Autodesk Inventor part; units mm, degrees
ref_plane "YZ Plane" through (0, 0, 0) normal (1, 0, 0) x (0, 1, 0)
ref_plane "XZ Plane" through (0, 0, 0) normal (0, 1, 0) x (-1, 0, 0)
ref_plane "XY Plane" through (0, 0, 0) normal (0, 0, 1) x (1, 0, 0)
sketch "Sketch1" plane through (0, 0, 0) normal (0, 1, 0) x (-1, 0, 0)
  line L0 (-10, -55) -> (-160, -55)
  line L1 (-160, -55) -> (-160, -45)
  line L2 (-160, -45) -> (-10, -45)
  line L3 (-10, -45) -> (-10, -55)
  line L4 (10, -55) -> (80, -55)
  line L5 (80, -55) -> (80, -90)
  line L6 (80, -90) -> (110, -90)
  line L7 (110, -90) -> (110, -10)
  line L8 (110, -10) -> (80, -10)
  line L9 (80, -10) -> (80, -45)
  line L10 (80, -45) -> (10, -45)
  line L11 (10, -45) -> (10, -55)
  line L12 (0, -122.2654) -> (0, -189.4683)
  line L13 (-10, 55) -> (-10, 45)
  line L14 (10, 55) -> (10, 45)
  line L15 (80, 10) -> (110, 10)
  line L16 (10, 45) -> (80, 45)
  line L17 (80, 45) -> (80, 10)
  line L18 (80, 55) -> (10, 55)
  line L19 (80, 90) -> (80, 55)
  line L20 (110, 10) -> (110, 90)
  line L21 (110, 90) -> (80, 90)
  line L22 (-160, 55) -> (-10, 55)
  line L23 (-160, 45) -> (-160, 55)
  line L24 (-10, 45) -> (-160, 45)
  point P0 (0, 0)
  dimension "d0" = 10
  dimension "d1" = 80
  dimension "d2" = 10
  dimension "d4" = 30
  dimension "d5" = 30
  dimension "d6" = 35
  dimension "d7" = 35
  dimension "d8" = 45
  dimension "d9" = 10
  dimension "d10" = 10
  dimension "d11" = 150
  dimension "d12" = 100
  dimension "d13" = 0
  dimension "d16" = 100
extrude "Extrusion1" add sketch "Sketch1" along normal blind 50
sketch "Sketch2" plane through (160, 0, 55) normal (1, 0, 0) x (0, 0, -1)
  line L0 (2.5, 40) -> (7.5, 40)
  line L1 (7.5, 40) -> (7.5, 35)
  line L2 (7.5, 35) -> (2.5, 35)
  line L3 (2.5, 35) -> (2.5, 40)
  line L4 (0, 50) -> (10, 50)
  line L5 (10, 0) -> (10, 50)
  line L6 (2.5, 15) -> (7.5, 15)
  line L7 (7.5, 15) -> (7.5, 10)
  line L8 (7.5, 10) -> (2.5, 10)
  line L9 (2.5, 10) -> (2.5, 15)
  line L10 (102.5, 40) -> (107.5, 40)
  line L11 (107.5, 40) -> (107.5, 35)
  line L12 (107.5, 35) -> (102.5, 35)
  line L13 (102.5, 35) -> (102.5, 40)
  line L14 (102.5, 15) -> (107.5, 15)
  line L15 (107.5, 15) -> (107.5, 10)
  line L16 (107.5, 10) -> (102.5, 10)
  line L17 (102.5, 10) -> (102.5, 15)
  point P0 (55, 0)
  dimension "d23" = 10
  dimension "d24" = 5
  dimension "d25" = 2.5
  dimension "d26" = 5
  dimension "d29" = 25
  dimension "d32" = 100
extrude "Extrusion2" cut sketch "Sketch2" against normal blind 200
sketch "Sketch3" plane through (0, 50, 0) normal (0, 1, 0) x (1, 0, 0)
  line L0 (-105, -20) -> (-85, -20)
  line L1 (-85, -20) -> (-85, -30)
  line L2 (-85, -30) -> (-105, -30)
  line L3 (-105, -30) -> (-105, -20)
  line L4 (-110, -10) -> (-110, -90)
  line L5 (-105, -70) -> (-85, -70)
  line L6 (-85, -70) -> (-85, -80)
  line L7 (-85, -80) -> (-105, -80)
  line L8 (-105, -80) -> (-105, -70)
  line L9 (-105, 80) -> (-85, 80)
  line L10 (-85, 80) -> (-85, 70)
  line L11 (-85, 70) -> (-105, 70)
  line L12 (-105, 70) -> (-105, 80)
  line L13 (-105, 30) -> (-85, 30)
  line L14 (-85, 30) -> (-85, 20)
  line L15 (-85, 20) -> (-105, 20)
  line L16 (-105, 20) -> (-105, 30)
  point P0 (0, 0)
  dimension "d37" = 20
  dimension "d38" = 10
  dimension "d39" = 20
  dimension "d40" = 85
  dimension "d43" = 50
  dimension "d46" = 100
extrude "Extrusion3" add sketch "Sketch3" along normal blind 8
sketch "Sketch4" plane through (0, 0, 0) normal (0, -1, 0) x (1, 0, 0)
  line L0 (-105, -70) -> (-85, -70)
  line L1 (-85, -70) -> (-85, -80)
  line L2 (-85, -80) -> (-105, -80)
  line L3 (-105, -80) -> (-105, -70)
  line L4 (-105, -20) -> (-85, -20)
  line L5 (-85, -20) -> (-85, -30)
  line L6 (-85, -30) -> (-105, -30)
  line L7 (-105, -30) -> (-105, -20)
  line L8 (-105, 30) -> (-85, 30)
  line L9 (-85, 30) -> (-85, 20)
  line L10 (-85, 20) -> (-105, 20)
  line L11 (-105, 20) -> (-105, 30)
  line L12 (-105, 80) -> (-85, 80)
  line L13 (-85, 80) -> (-85, 70)
  line L14 (-85, 70) -> (-105, 70)
  line L15 (-105, 70) -> (-105, 80)
  line L16 (-85, 80) -> (-105, 80)
  line L17 (-105, 80) -> (-105, 70)
  line L18 (-105, 70) -> (-85, 70)
  line L19 (-85, 70) -> (-85, 80)
  line L20 (-85, 30) -> (-105, 30)
  line L21 (-105, 30) -> (-105, 20)
  line L22 (-105, 20) -> (-85, 20)
  line L23 (-85, 20) -> (-85, 30)
  line L24 (-85, -20) -> (-105, -20)
  line L25 (-105, -20) -> (-105, -30)
  line L26 (-105, -30) -> (-85, -30)
  line L27 (-85, -30) -> (-85, -20)
  line L28 (-85, -70) -> (-105, -70)
  line L29 (-105, -70) -> (-105, -80)
  line L30 (-105, -80) -> (-85, -80)
  line L31 (-85, -80) -> (-85, -70)
  point P0 (0, 0)
extrude "Extrusion4" cut sketch "Sketch4" against normal blind 10
sketch "Sketch5" plane through (10, 0, 55) normal (0, 0, 1) x (1, 0, 0)
  line L0 (0, 0) -> (0, 50)
  line L1 (0, 50) -> (150, 50)
  line L2 (150, 0) -> (150, 50)
  line L3 (0, 0) -> (150, 0)
  line L4 (0, 35) -> (0, 40)
  line L5 (150, 35) -> (0, 35)
  line L6 (150, 40) -> (150, 35)
  line L7 (150, 40) -> (0, 40)
  line L8 (0, 10) -> (0, 15)
  line L9 (150, 10) -> (0, 10)
  line L10 (150, 15) -> (150, 10)
  line L11 (150, 15) -> (0, 15)
  line L12 (10, 40) -> (140, 40)
  line L13 (140, 40) -> (140, 35)
  line L14 (140, 35) -> (10, 35)
  line L15 (10, 35) -> (10, 40)
  line L16 (10, 15) -> (140, 15)
  line L17 (140, 15) -> (140, 10)
  line L18 (140, 10) -> (10, 10)
  line L19 (10, 10) -> (10, 15)
  point P0 (-10, 0)
  point P1 (10, 10)
  dimension "d53" = 10
  dimension "d54" = 10
  dimension "d55" = 10
  dimension "d56" = 10
extrude "Extrusion5" add sketch "Sketch5" against normal blind 10 contours L19 L11 L17 L9 | L15 L7 L13 L5
sketch "Sketch6" plane through (160, 0, -55) normal (0, 0, -1) x (-1, 0, 0)
  line L0 (150, 40) -> (150, 35)
  line L1 (0, 40) -> (150, 40)
  line L2 (0, 35) -> (0, 40)
  line L3 (0, 35) -> (150, 35)
  line L4 (150, 15) -> (150, 10)
  line L5 (0, 15) -> (150, 15)
  line L6 (0, 10) -> (0, 15)
  line L7 (0, 10) -> (150, 10)
  line L8 (10, 40) -> (140, 40)
  line L9 (140, 40) -> (140, 35)
  line L10 (140, 35) -> (10, 35)
  line L11 (10, 35) -> (10, 40)
  line L12 (10, 15) -> (140, 15)
  line L13 (140, 15) -> (140, 10)
  line L14 (140, 10) -> (10, 10)
  line L15 (10, 10) -> (10, 15)
  point P0 (160, 0)
  point P1 (140, 37.5)
  point P2 (10, 10)
  dimension "d59" = 10
  dimension "d60" = 10
  dimension "d61" = 10
  dimension "d62" = 10
extrude "Extrusion6" add sketch "Sketch6" against normal blind 10 contours L9 L3 L11 L1 | L13 L7 L15 L5
sketch "Sketch7" plane through (0, 58, 0) normal (0, 1, 0) x (1, 0, 0)
  line L0 (-105, -80) -> (-85, -80)
  line L1 (-85, -80) -> (-85, -70)
  line L2 (-85, -70) -> (-105, -70)
  line L3 (-105, -70) -> (-105, -80)
  line L4 (-105, -30) -> (-85, -30)
  line L5 (-85, -30) -> (-85, -20)
  line L6 (-85, -20) -> (-105, -20)
  line L7 (-105, -20) -> (-105, -30)
  line L8 (-105, 20) -> (-85, 20)
  line L9 (-85, 20) -> (-85, 30)
  line L10 (-85, 30) -> (-105, 30)
  line L11 (-105, 30) -> (-105, 20)
  line L12 (-105, 70) -> (-85, 70)
  line L13 (-85, 70) -> (-85, 80)
  line L14 (-85, 80) -> (-105, 80)
  line L15 (-105, 80) -> (-105, 70)
  line L16 (-104, -79) -> (-86, -79)
  line L17 (-86, -79) -> (-86, -71)
  line L18 (-86, -71) -> (-104, -71)
  line L19 (-104, -71) -> (-104, -79)
  line L20 (-86, -21) -> (-104, -21)
  line L21 (-104, -21) -> (-104, -29)
  line L22 (-104, -29) -> (-86, -29)
  line L23 (-86, -29) -> (-86, -21)
  line L24 (-86, 29) -> (-104, 29)
  line L25 (-104, 29) -> (-104, 21)
  line L26 (-104, 21) -> (-86, 21)
  line L27 (-86, 21) -> (-86, 29)
  line L28 (-86, 79) -> (-104, 79)
  line L29 (-104, 79) -> (-104, 71)
  line L30 (-104, 71) -> (-86, 71)
  line L31 (-86, 71) -> (-86, 79)
  line L32 (-105, -80) -> (-85, -80)
  line L33 (-85, -80) -> (-85, -70)
  line L34 (-85, -70) -> (-105, -70)
  line L35 (-105, -70) -> (-105, -80)
  line L36 (-105, -30) -> (-85, -30)
  line L37 (-85, -30) -> (-85, -20)
  line L38 (-85, -20) -> (-105, -20)
  line L39 (-105, -20) -> (-105, -30)
  line L40 (-105, 20) -> (-85, 20)
  line L41 (-85, 20) -> (-85, 30)
  line L42 (-85, 30) -> (-105, 30)
  line L43 (-105, 30) -> (-105, 20)
  line L44 (-105, 70) -> (-85, 70)
  line L45 (-85, 70) -> (-85, 80)
  line L46 (-85, 80) -> (-105, 80)
  line L47 (-105, 80) -> (-105, 70)
  point P0 (0, 0)
  dimension "d65" = 1
  dimension "d66" = 1
  dimension "d67" = 1
  dimension "d68" = 1
  dimension "d71" = 50
  dimension "d74" = 100
extrude "Extrusion7" cut sketch "Sketch7" against normal blind 8
sketch "Sketch8" plane through (-80, 0, 55) normal (0, 0, 1) x (1, 0, 0)
  line L0 (70, 40) -> (70, 35)
  line L1 (70, 40) -> (40, 40)
  line L2 (40, 40) -> (40, 35)
  line L3 (70, 35) -> (40, 35)
  line L4 (70, 15) -> (70, 10)
  line L5 (70, 15) -> (40, 15)
  line L6 (40, 15) -> (40, 10)
  line L7 (70, 10) -> (40, 10)
  line L8 (40, 40) -> (60, 40)
  line L9 (60, 40) -> (60, 35)
  line L10 (60, 35) -> (40, 35)
  line L11 (40, 35) -> (40, 40)
  line L12 (40, 15) -> (60, 15)
  line L13 (60, 15) -> (60, 10)
  line L14 (60, 10) -> (40, 10)
  line L15 (40, 10) -> (40, 15)
  point P0 (80, 0)
  point P1 (60, 15)
  point P2 (60, 40)
  dimension "d79" = 10
  dimension "d80" = 10
extrude "Extrusion8" add sketch "Sketch8" against normal blind 10 contours L9 L3 L2 L1 | L13 L7 L6 L5
sketch "Sketch9" plane through (-10, 0, -55) normal (0, 0, -1) x (-1, 0, 0)
  line L0 (0, 35) -> (0, 40)
  line L1 (0, 35) -> (30, 35)
  line L2 (30, 35) -> (30, 40)
  line L3 (0, 40) -> (30, 40)
  line L4 (0, 10) -> (0, 15)
  line L5 (0, 10) -> (30, 10)
  line L6 (30, 10) -> (30, 15)
  line L7 (0, 15) -> (30, 15)
  line L8 (30, 40) -> (10, 40)
  line L9 (10, 40) -> (10, 10)
  line L10 (10, 10) -> (30, 10)
  line L11 (30, 10) -> (30, 40)
  point P0 (-10, 0)
  point P1 (0, 37.5)
  dimension "d83" = 10
extrude "Extrusion9" add sketch "Sketch9" against normal blind 10 contours L9 L3 L2 L1 | L1 L11 L7 L9 | L7 L6 L5 L9
sketch "Sketch10" plane through (0, 58, 0) normal (0, 1, 0) x (1, 0, 0)
  line L0 (-140, 100) -> (-140, 0)
  line L1 (-140, 0) -> (0, 0)
  line L2 (0, 0) -> (0, -100)
  line L3 (0, -100) -> (180, -100)
  line L4 (180, -100) -> (180, 100)
  line L5 (180, 100) -> (-140, 100)
  dimension "d86" = 100
  dimension "d87" = 320
  dimension "d88" = 200
  dimension "d89" = 180
extrude "Extrusion10" cut sketch "Sketch10" against normal through all
properties part number "Hurdle Split"
Could you check a few things on this model? Use its own coordinates, in mm. A direction names the side the tool comes from. Coordinates: 2 decimals unless noted, no trailing zeros. Order: outer loops, then holes, each group sorted by start corner. A loop starts at its lowest first (then second) coordinate and runs counter-clockwise, first axis right, second up.
Q1. Suppose I cut it at C-C on x = -90. Please give me the cut outline in (y, z).
Q2. Please list where these lines run through material, in increasing order: L1, parallel to Z at x = -91.5, y = 8; L2, parallel to X at y = 13.5, z = 82.5; L3, parallel to X at y = 11, z = 50.
Q3. Suppose I cut it at B-B on y = 43. Please give me the cut outline in (x, z).
Q4. Thinking about a two-plate mould opening in Z: for faces 1 (the flat face through (-15, 13, 47.5)), 2 (the flat face through (-95, 25, 10)), 3 (the flat face through (-104, 54, 25)), which applies, released by +Z, released by -Z, zero draft, split by the parting line, or undercut?
Q5. Suppose I cut it at A-A on y = 53. Please give me the cut outline in (x, z).
Q6. Which directions (+Z, -Z, +X, -X, +Y, -Y) give clear straight access to the entire face, cutting with the end or side of a thin tool? Please do faces 4 (the flat face through (-95, 5, 30)), 5 (the flat face through (-104, 54, 75)), 6 (the flat face through (-95, 54, 29)).
Q7. Suppose I cut it at D-D on z = 36.5. Please give me the cut outline in (x, y), and give its area (3 significant figures).
Q8. Will these pins go through, and if not, where does the flat tip stop? pin 1 (6 mm diameter, centred on x = -34.5, y = 42, fed in from -Z); pin 2 (3 mm diameter, centred on y = 6.5, z = 75, fed in from +X); pin 3 (2.5 mm diameter, centred on y = 13, z = 49.5, fed in from +X).
Answer:
1. outline: (0, 10) - (50, 10) - (50, 21) - (58, 21) - (58, 29) - (50, 29) - (50, 71) - (58, 71) - (58, 79) - (50, 79) - (50, 90) - (0, 90) - (0, 80) - (10, 80) - (10, 70) - (0, 70) - (0, 30) - (10, 30) - (10, 20) - (0, 20) - close
2. L1: z = 10 to 20, 30 to 70, 80 to 90
2. L2: x = -110 to -80
2. L3: x = -110 to -20
3. outline: (-110, 10) - (-80, 10) - (-80, 45) - (-10, 45) - (-10, 55) - (-80, 55) - (-80, 90) - (-110, 90) - close
4. face 1: undercut
4. face 2: released by -Z
4. face 3: zero draft
5. outline: (-104, 21) - (-86, 21) - (-86, 29) - (-104, 29) - close; (-104, 71) - (-86, 71) - (-86, 79) - (-104, 79) - close
6. face 4: -Y
6. face 5: +Z, -Z, -X, +Y
6. face 6: +X, -X, +Y
7. outline: (-110, 0) - (-80, 0) - (-80, 50) - (-110, 50) - close
7. area: 1,500 mm2
8. pin 1: stops at z = 45
8. pin 2: stops at x = -80
8. pin 3: stops at x = -20
